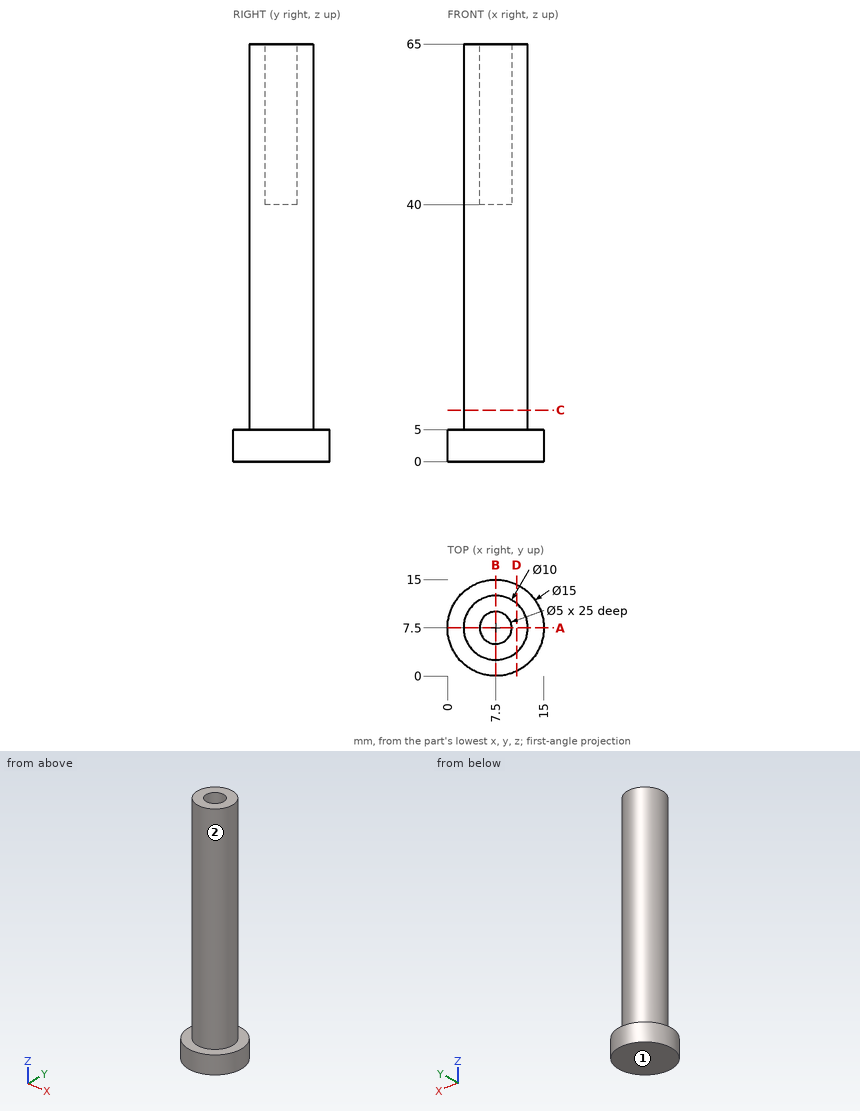
Answer from the drawing. Dimensions are ordinates in mm from the lowest x, y and z of the part. A direction names the side the tool comes from. Round coordinates to 2 decimals unless told otherwise and drop trailing zeros. Write each loop counter-clockwise with the first axis right and the second up, starting at its lowest first coordinate (ties: lowest second). Pieces come first, ordered by that corner, then holes.
1. Given pin 1 Ø5 at (y, z) = (12, 13) entering from +X; pin 2 Ø6 at (x, y) = (7, 6.5) entering from -Z; pin 3 Ø4 at (x, y) = (7.5, 7.5) entering from +Z; pin 4 Ø1.5 at (y, z) = (3, 27.5) entering from -X, each flat-ended and moving along its own axis, determine where each tip first touches the part or whether it passes through.
2. The part is cut by section C-C, the plane z = 8. Determine the outline of the cut face in (x, y), then the cut area to 3 significant figures.
3. The part is cut by section A-A, the plane y = 7.5. Determine the outline of the cut face in (x, z), then the cut area to 3 significant figures.
4. Which of the six approach directions +Z, -Z, +X, -X, +Y, -Y give full straight-line access (tool end or side, diameter ignored) to the marked faces 1 and 2?
5. The part is cut by section D-D, the plane x = 10.75. Determine the outline of the cut face in (y, z), then the cut area to 3 significant figures.
6. Straight lines are drawn through the part: L1, parallel to Y at x = 7.5, z = 53.75; L2, parallel to Z at x = 10.5, y = 12; L3, parallel to Y at x = 9.25, z = 50. For each, find the intervals that lie inside material, in ascending order.
Values:
1. pin 1: stops at x = 12.08
1. pin 2: stops at z = 0
1. pin 3: stops at z = 40
1. pin 4: stops at x = 4.19
2. outline: circle Ø10 at (7.5, 7.5)
2. area: 78.5 mm2
3. outline: (0, 0) - (15, 0) - (15, 5) - (12.5, 5) - (12.5, 65) - (10, 65) - (10, 40) - (5, 40) - (5, 65) - (2.5, 65) - (2.5, 5) - (0, 5) - close
3. area: 550 mm2
4. face 1: -Z, +X, -X, +Y, -Y
4. face 2: +Z
5. outline: (0.74, 0) - (14.26, 0) - (14.26, 5) - (11.3, 5) - (11.3, 65) - (3.7, 65) - (3.7, 5) - (0.74, 5) - close
5. area: 524 mm2
6. L1: y = 2.5 to 5, 10 to 12.5
6. L2: z = 0 to 5
6. L3: y = 2.82 to 5.71, 9.29 to 12.18
